Verification items for this drawing (mm, ordinates from the low corner). Round coordinates to 2 decimals unless told otherwise and drop trailing zeros. Write each loop counter-clockwise with the first axis right and the second up, starting at its lowest first coordinate (ties: lowest second). Pieces come first, ordered by that corner, then holes.
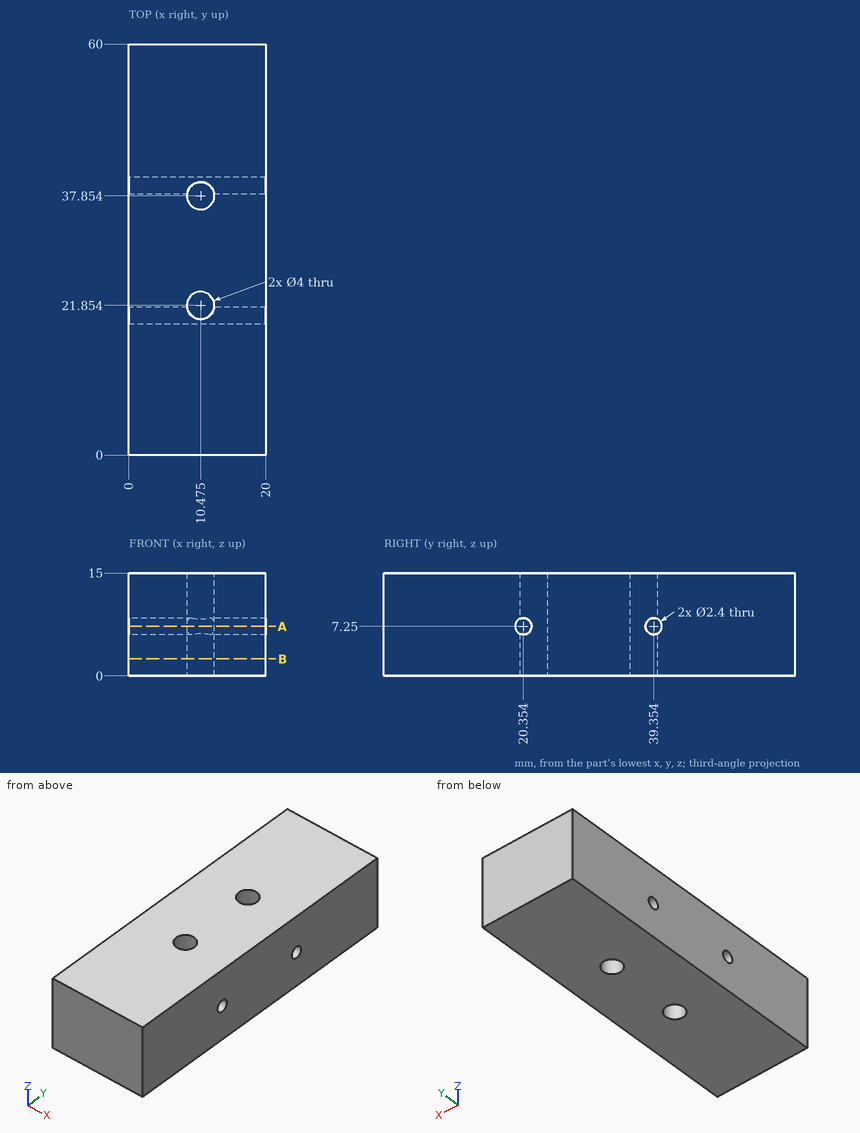
1. Depth check by flat-ended pin: pin 1 Ø4 at (y, z) = (39.35, 7.25) entering from -X; pin 2 Ø1.4 at (y, z) = (20.35, 7.25) entering from +X. Enter the tip coordinate at first touch or a pass-through.
2. Section check B-B (z = 2.5). Record the cut outline in (x, y) (3 decimals).
3. Scan lines: line 1 along Y through (x, z) = (1.5, 7.5); line 2 along Y through (x, z) = (6.75, 8); line 3 along Z through (x, y) = (14.5, 39). Record each from-to range of solid material in increasing order.
4. Section check A-A (z = 7.25). Record the cut outline in (x, y) (1 decimal).
Results below:
1. pin 1: stops at x = 0
1. pin 2: passes through
2. outline: (0, 0) - (20, 0) - (20, 60) - (0, 60) - close; hole circle Ø4 at (10.475, 21.854); hole circle Ø4 at (10.475, 37.854)
3. line 1: y = 0 to 19.18, 21.53 to 38.18, 40.53 to 60
3. line 2: y = 0 to 19.42, 21.29 to 38.42, 40.29 to 60
3. line 3: z = 0 to 6.1, 8.4 to 15
4. outline: (0, 0) - (20, 0) - (20, 19.2) - (0, 19.2) - close; (0, 21.6) - (8.5, 21.6) arc R2 cw (long way) to (12.5, 21.6) - (20, 21.6) - (20, 38.2) - (12.5, 38.2) arc R2 cw (long way) to (8.5, 38.2) - (0, 38.2) - close; (0, 40.6) - (20, 40.6) - (20, 60) - (0, 60) - close
